Here's how the part is built. I have some questions about the finished solid (model axes, mm). Face numbers are marked on the shaded views. A direction names the side the tool comes from. Coordinates: 2 decimals unless noted, no trailing zeros. Write each loop counter-clockwise with the first axis right and the second up, starting at its lowest first coordinate (ties: lowest second). Pieces come first, ordered by that corner, then holes. Notation, with made-up numbers: (1, 48) -> (5, 48) arc R27 cw to (5, 74) -> close; hole circle Ø5 at (-28.75, -11). An arc over 180 degrees is marked (long way). Use a Markdown table: item, result. Add a question column.
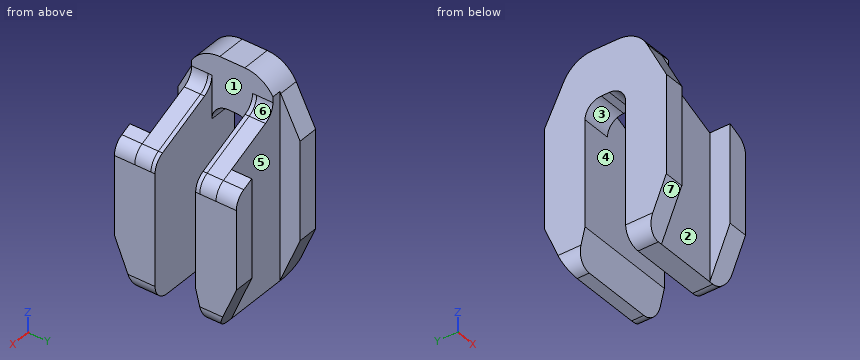
Autodesk Inventor part; units mm, degrees
ref_plane "YZ Plane" through (0, 0, 0) normal (1, 0, 0) x (0, 1, 0)
ref_plane "XZ Plane" through (0, 0, 0) normal (0, 1, 0) x (-1, 0, 0)
ref_plane "XY Plane" through (0, 0, 0) normal (0, 0, 1) x (1, 0, 0)
sketch "Sketch1" plane through (0, 0, 0) normal (0, 0, 1) x (1, 0, 0)
  line L0 (-4.78, -2.9) -> (4.78, -2.9)
  line L1 (6.35, 2.9) -> (-6.35, 2.9)
  line L2 (-4.78, -2.9) -> (-5.08, -2.9)
  line L3 (-6.35, -2.9) -> (-5.08, -2.9)
  line L4 (-6.35, 2.9) -> (-6.35, -2.9)
  line L5 (5.08, -2.9) -> (4.78, -2.9)
  line L6 (5.08, -2.9) -> (6.35, -2.9)
  line L7 (6.35, 3) -> (-6.45, 3)
  line L8 (-6.45, 3) -> (-6.45, -3)
  line L9 (-6.45, -3) -> (-5.08, -3)
  line L10 (-5.08, -3) -> (-4.78, -3)
  line L11 (-4.78, -3) -> (4.78, -3)
  line L12 (4.78, -3) -> (5.08, -3)
  line L13 (5.08, -3) -> (6.35, -3)
  line L14 (6.35, 5) -> (-8.45, 5)
  line L15 (-8.45, 5) -> (-8.45, -5)
  line L16 (-8.45, -5) -> (-5.08, -5)
  line L17 (-5.08, -5) -> (-4.78, -5)
  line L18 (-4.78, -5) -> (4.78, -5)
  line L19 (4.78, -5) -> (5.08, -5)
  line L20 (5.08, -5) -> (6.35, -5)
  line L21 (6.35, 3) -> (6.35, 5)
  line L22 (6.35, -3) -> (6.35, -5)
  point P0 (0, 0)
extrude "Extrusion1" add sketch "Sketch1" against normal blind 2
sketch "Sketch2" plane through (-8.45, -5, 0) normal (0, -1, 0) x (1, 0, 0)
  line L0 (2.1, -8) -> (2.1, -11.17)
  line L1 (0, 0) -> (14.8, 0)
  line L2 (2.1, -8) -> (3.37, -8)
  line L3 (14.8, 0) -> (14.8, -2)
  line L4 (2, 0) -> (14.8, 0)
  line L5 (2, 0) -> (14.8, 0)
  line L6 (14.8, 0) -> (14.8, -8)
  line L7 (14.8, -8) -> (2, -8)
  line L8 (2, -8) -> (2, 0)
  point P0 (8.45, 0)
extrude "Extrusion2" add sketch "Sketch2" against normal up to surface (2 mm away)
sketch "Sketch3" plane through (-8.45, 5, 0) normal (0, 1, 0) x (1, 0, 0)
  line L0 (0, 0) -> (14.8, 0)
  line L1 (0, 0) -> (0, 2)
  line L2 (2, 2) -> (0, 2)
  line L3 (2, 2) -> (2, 8)
  line L4 (2, 8) -> (14.8, 8)
  line L5 (14.8, 0) -> (14.8, 8)
  point P0 (8.45, 0)
extrude "Extrusion3" add sketch "Sketch3" against normal up to surface (2 mm away)
sketch "Sketch4" plane through (-8.45, -5, 0) normal (0, -1, 0) x (1, 0, 0)
  line L0 (2, -2) -> (2, -8)
  line L1 (0, 0) -> (14.8, 0)
  line L2 (3.67, -0.6428) -> (3.67, -14.175)
  line L3 (5.61, -0.6428) -> (5.61, -14.175)
  line L4 (2, -2) -> (5.61, -2)
  line L5 (5.61, -2) -> (5.61, 4)
  line L6 (5.61, 4) -> (2, 4)
  line L7 (2, 4) -> (2, -2)
  point P0 (8.45, 0)
  point P1 (2, 0)
  point P2 (5.61, 0)
  dimension "d8" = 6
extrude "Extrusion4" add sketch "Sketch4" against normal up to surface (10 mm away) contours L7 L6 L5 L1
sketch "Sketch5" plane through (-8.45, -5, -2) normal (0, -1, 0) x (1, 0, 0)
  line L0 (0, 2) -> (0, 0)
  line L1 (0, 2) -> (2, 2)
  line L2 (2, 0) -> (0, 0)
  line L3 (0, 2) -> (2, 2)
  line L4 (2, 2) -> (2, 0)
  line L5 (2, 0) -> (0, 0)
  line L6 (0, 0) -> (0, 2)
  point P0 (8.45, 2)
extrude "Extrusion5" cut sketch "Sketch5" against normal through all
sketch "Sketch6" plane through (-6.45, -5, -8) normal (0, -1, 0) x (1, 0, 0)
  line L0 (3.61, 8) -> (3.61, 12)
  line L1 (3.61, 8) -> (12.8, 8)
  line L2 (3.61, 12) -> (12.8, 8)
  point P0 (6.45, 8)
extrude "Extrusion6" add sketch "Sketch6" against normal up to surface (2 mm away)
sketch "Sketch7" plane through (-6.45, 5, -8) normal (0, 1, 0) x (1, 0, 0)
  line L0 (12.8, -8) -> (3.61, -12)
  line L1 (12.8, -8) -> (3.61, -8)
  line L2 (3.61, -8) -> (3.61, -12)
  point P0 (6.45, -8)
extrude "Extrusion7" add sketch "Sketch7" against normal up to surface (2 mm away)
sketch "Sketch8" plane through (-2.84, -3, 0) normal (1, 0, 0) x (0, 0, -1)
  line L0 (0, 6) -> (-4, 6)
  line L1 (-4, 0) -> (-4, 6)
  line L2 (-4, 0) -> (0, 0)
  line L3 (0, 0) -> (0, 6)
  line L4 (-4, 0) -> (0, 0)
  line L5 (-2, 0) -> (-2, 6)
  point P0 (0, 3)
  point P1 (-2, 0)
extrude "Extrusion8" cut sketch "Sketch8" against normal blind 10 contours L3 L2 L5 L0
sketch "Sketch9" plane through (-6.45, -5, 4) normal (0, 0, 1) x (1, 0, 0)
  line L0 (0, 8) -> (0, 2)
  line L1 (3.61, 10) -> (0, 10)
  line L2 (0, 0) -> (0, 10)
  line L3 (3.61, 0) -> (0, 0)
  line L4 (3.61, 0) -> (3.61, 2)
  line L5 (3.61, 2) -> (3.61, 8)
  line L6 (3.61, 8) -> (3.61, 10)
  point P0 (6.45, 5)
  point P1 (0, 2)
extrude "Extrusion9" add sketch "Sketch9" along normal blind 4
fillet "Fillet1" radius 2 4 edges at (-2.84, 4, 4) (-2.84, -4, 4) (6.35, 4, 0) (6.35, -4, 0)
sketch "Sketch10" plane through (6.35, -5, -8) normal (0, 0, -1) x (-1, 0, 0)
  line L0 (12.8, 2) -> (0, 2)
  line L1 (0, 0) -> (0, 2)
  line L2 (12.8, 0) -> (0, 0)
  line L3 (12.8, 0) -> (12.8, 2)
  line L4 (0, 8) -> (12.8, 8)
  line L5 (12.8, 10) -> (12.8, 8)
  line L6 (0, 10) -> (12.8, 10)
  line L7 (0, 10) -> (0, 8)
  point P0 (6.35, 5)
extrude "Extrusion10" add sketch "Sketch10" along normal blind 4
sketch "Sketch11" plane through (-6.45, 3, 2) normal (0, -1, 0) x (1, 0, 0)
  arc A0 (12.8, -3.3107) -> (11.5982, -1.4769) centre (10.8, -3.3107) ccw
  line L0 (4.8118, 1.4769) -> (11.5982, -1.4769)
  arc A1 (3.61, 3.3107) -> (4.8118, 1.4769) centre (5.61, 3.3107) ccw
  line L1 (3.61, 0) -> (3.61, 3.3107)
  line L2 (3.61, 0) -> (0, 0)
  line L3 (0, 0) -> (0, -14)
  line L4 (12.8, -14) -> (0, -14)
  line L5 (12.8, -3.3107) -> (12.8, -14)
  point P0 (6.45, -2)
extrude "Extrusion11" add sketch "Sketch11" along normal blind 0.5
sketch "Sketch12" plane through (-6.45, -3, 2) normal (0, 1, 0) x (1, 0, 0)
  arc A0 (11.5982, 1.4769) -> (12.8, 3.3107) centre (10.8, 3.3107) ccw
  line L0 (12.8, 3.3107) -> (12.8, 14)
  line L1 (0, 14) -> (12.8, 14)
  line L2 (0, 0) -> (0, 14)
  line L3 (3.61, 0) -> (0, 0)
  line L4 (3.61, -3.3107) -> (3.61, 0)
  arc A1 (4.8118, -1.4769) -> (3.61, -3.3107) centre (5.61, -3.3107) ccw
  line L5 (11.5982, 1.4769) -> (4.8118, -1.4769)
  point P0 (6.45, 2)
extrude "Extrusion12" add sketch "Sketch12" along normal blind 0.5
fillet "Fillet3" radius 2 2 edges at (-4.645, -2.5, 2) (-4.645, 2.5, 2)
sketch "Sketch14" plane through (6.35, -5, -12) normal (0, 0, -1) x (-1, 0, 0)
  line L0 (0, 0) -> (0, 2.5)
  line L1 (0, 0) -> (12.8, 0)
  line L2 (12.8, 0) -> (12.8, 2.5)
  line L3 (0, 2.5) -> (12.8, 2.5)
  line L4 (12.8, 10) -> (12.8, 7.5)
  line L5 (12.8, 10) -> (0, 10)
  line L6 (0, 10) -> (0, 7.5)
  line L7 (12.8, 7.5) -> (0, 7.5)
  point P0 (6.35, 5)
extrude "Extrusion13" add sketch "Sketch14" along normal blind 5
sketch "Sketch15" plane through (6.35, -5, -17) normal (0, 0, -1) x (-1, 0, 0)
  line L0 (12.8, 2.5) -> (0, 2.5)
  line L1 (0, 2.5) -> (0, 0)
  line L2 (0, 0) -> (12.8, 0)
  line L3 (12.8, 0) -> (12.8, 2.5)
  line L4 (0, 7.5) -> (12.8, 7.5)
  line L5 (12.8, 7.5) -> (12.8, 10)
  line L6 (12.8, 10) -> (0, 10)
  line L7 (0, 10) -> (0, 7.5)
  line L8 (12.8, 0) -> (10.3, 0)
  line L9 (10.3, 0) -> (10.3, -2.5)
  line L10 (10.3, -2.5) -> (12.8, -2.5)
  line L11 (12.8, -2.5) -> (12.8, 0)
  line L12 (12.8, 10) -> (10.3, 10)
  line L13 (10.3, 10) -> (10.3, 12.5)
  line L14 (10.3, 12.5) -> (12.8, 12.5)
  line L15 (12.8, 12.5) -> (12.8, 10)
  line L16 (0, 10) -> (2.5, 10)
  line L17 (2.5, 10) -> (2.5, 12.5)
  line L18 (2.5, 12.5) -> (0, 12.5)
  line L19 (0, 12.5) -> (0, 10)
  line L20 (0, 0) -> (2.5, 0)
  line L21 (2.5, 0) -> (2.5, -2.5)
  line L22 (2.5, -2.5) -> (0, -2.5)
  line L23 (0, -2.5) -> (0, 0)
  point P0 (6.35, 5)
  point P1 (2.5, 10)
  point P2 (2.5, 0)
  dimension "d39" = 2.5
  dimension "d40" = 2.5
  dimension "d41" = 2.5
  dimension "d42" = 2.5
  dimension "d43" = 2.5
  dimension "d44" = 2.5
  dimension "d45" = 2.5
  dimension "d46" = 2.5
extrude "Extrusion14" add sketch "Sketch15" against normal up to surface (25 mm away) contours L11 L10 L9 L2 | L2 L21 L22 L23 | L19 L18 L17 L6 | L6 L13 L14 L15
sketch "Sketch16" plane through (3.85, 5, 8) normal (0, -1, 0) x (1, 0, 0)
  line L0 (0, -6.9119) -> (1.2982, -7.4769)
  arc A0 (2.5, -9.3107) -> (1.2982, -7.4769) centre (0.5, -9.3107) ccw
  line L1 (2.5, -9.3107) -> (2.5, 0)
  line L2 (2.5, 0) -> (0, 0)
  line L3 (0, -6.9119) -> (0, 0)
  point P0 (-3.85, -8)
extrude "Extrusion15" cut sketch "Sketch16" along normal mid plane 31
fillet "Fillet5" radius 2 4 edges at (6.35, 5, -17) (-6.45, 5, -17) (6.35, -5, -17) (-6.45, -5, -17)
chamfer "Chamfer3" distance 2.5 angle 45 2 edges at (-5.2, -7.5, 8) (-5.2, 7.5, 8)
sketch "Sketch17" plane through (-6.45, 2.5, -15) normal (-1, 0, 0) x (0, 0, 1)
  line L0 (-2, 5) -> (-2, 0)
  line L1 (-2, 5) -> (0, 5)
  line L2 (0, 5) -> (20.5, 5)
  line L3 (0, 0) -> (-2, 0)
  line L4 (15, 0) -> (0, 0)
  line L5 (-2, 0) -> (-2, 1)
  line L6 (-2, 0) -> (-2, 5)
  line L7 (-2, 0) -> (2, 0)
  line L8 (2, 0) -> (-2, 1)
  point P0 (15, -2.5)
  point P1 (-2, 1)
  dimension "d55" = 1
  dimension "d56" = 4
extrude "Extrusion16" cut sketch "Sketch17" against normal blind 31
sketch "Sketch18" plane through (-6.45, -7.5, -15) normal (-1, 0, 0) x (0, 0, 1)
  line L0 (16.0881, 12.5) -> (-2, 12.5)
  line L1 (0, 15) -> (20.5, 15)
  line L2 (-2, 2.5) -> (16.0881, 2.5)
  line L3 (0, 0) -> (20.5, 0)
  line L4 (-2, 15) -> (0, 15)
  line L5 (-2, 15) -> (-2, 11)
  line L6 (-2, 5) -> (-2, 0)
  line L7 (0, 0) -> (-2, 0)
  line L8 (-2, 0) -> (4, 0)
  line L9 (4, 0) -> (-2, 2.5)
  line L10 (-2, 15) -> (4, 15)
  line L11 (4, 15) -> (-2, 12.5)
  point P0 (15, 7.5)
  dimension "d59" = 6
  dimension "d60" = 6
extrude "Extrusion17" cut sketch "Sketch18" against normal through all
sketch "Sketch19" plane through (-6.45, -2.5, -15) normal (-1, 0, 0) x (0, 0, 1)
  line L0 (23, -2.5) -> (23, 7.5)
  line L1 (20.5, 10) -> (23, 7.5)
  line L2 (23, -2.5) -> (20.5, -5)
  line L3 (4, 10) -> (20.5, 10)
  line L4 (4, -5) -> (20.5, -5)
  line L5 (16.0881, -5) -> (16.0881, -2.5)
  line L6 (16.0881, 7.5) -> (16.0881, 10)
  line L7 (23, -2.5) -> (23, -1.5)
  line L8 (23, -1.5) -> (16.0881, -5)
  line L9 (23, 7.5) -> (23, 6.5)
  line L10 (23, 6.5) -> (16.0881, 10)
  point P0 (15, 2.5)
  dimension "d63" = 1
  dimension "d64" = 1
extrude "Extrusion18" cut sketch "Sketch19" against normal up to surface (3.61 mm away)
fillet "Fillet6" radius 4 2 edges at (-4.645, -4, 8) (-4.645, 4, 8)
properties part number "MolexClipper_vertical_3DPrint"
Q1. Thinking about a two-plate mould opening in Y: for the marked faces 4, 5, 6 and 7, which applies, released by +Y, released by -Y, zero draft, split by the parting line, or undercut?
Q2. Which directions (+Z, -Z, +X, -X, +Y, -Y) give clear straight access to the entire face, cutting with the end or side of a thin tool? Please do the marked faces 1, 2 and 3.
Q3. Suppose I cut it at B-B, the plane z = -6.25. Write out the boundary of the cut face in (x, y), and give its area (3 significant figures).
Q4. Please list where these lines run through material, in increasing order: line 1 (Y direction, x = 0.75, z = -3.25); line 2 (X direction, y = 5.5, z = -7); line 3 (Y direction, x = -4.75, z = -9.75).
Q5. Suppose I cut it at A-A, the plane x = 3.5. Write out the boundary of the cut face in (y, z), and give its area (3 significant figures).
Q6. Will these pins go through, and if not, where does the flat tip stop? pin 1 (2.5 mm diameter, centred on x = -1, z = -0.5, fed in from -Y); pin 2 (4 mm diameter, centred on x = 1.5, z = -1.5, fed in from +Y); pin 3 (1.5 mm diameter, centred on x = 0.5, y = -6, fed in from +Z).
Q7. Suppose I cut it at D-D, the plane z = -12. Write out the boundary of the cut face in (x, y).
Q8. Suppose I cut it at C-C, the plane y = -5.5. Write out the boundary of the cut face in (x, z), and give its area (3 significant figures).
Answer key:
| question | item | result |
|---|---|---|
| 1 | face 4 | undercut |
| 1 | face 5 | released by +Y |
| 1 | face 6 | zero draft |
| 1 | face 7 | released by -Y |
| 2 | face 1 | +Z, +X |
| 2 | face 2 | +Z, -Z, -Y |
| 2 | face 3 | -Z, +X, -X |
| 3 | outline | (-6.45, -7.5) -> (-3.95, -7.5) -> (-3.95, -5) -> (3.85, -5) -> (3.85, -7.5) -> (6.35, -7.5) -> (6.35, -2.5) -> (-6.45, -2.5) -> close; (-6.45, 2.5) -> (6.35, 2.5) -> (6.35, 7.5) -> (3.85, 7.5) -> (3.85, 5) -> (-3.95, 5) -> (-3.95, 7.5) -> (-6.45, 7.5) -> close |
| 3 | area | 89.0 mm^2 |
| 4 | line 1 | y = -5 to -2.5, 2.5 to 5 |
| 4 | line 2 | x = -6.45 to -3.95, 3.85 to 6.35 |
| 4 | line 3 | y = -7.5 to -2.5, 2.5 to 7.5 |
| 5 | outline | (-5, -17) -> (-2.5, -17) -> (-2.5, 1.24) -> (-5, 1.24) -> close; (2.5, -13) -> (3.5, -17) -> (5, -17) -> (5, 1.24) -> (2.5, 1.24) -> close |
| 5 | area | 89.2 mm^2 |
| 6 | pin 1 | stops at y = -5 |
| 6 | pin 2 | stops at y = 5 |
| 6 | pin 3 | passes through |
| 7 | outline | (-6.45, -7.08) -> (-3.95, -7.08) -> (-3.95, -5) -> (3.85, -5) -> (3.85, -7.08) -> (6.35, -7.08) -> (6.35, -2.5) -> (-6.45, -2.5) -> close; (-6.45, 2.5) -> (6.35, 2.5) -> (6.35, 7.08) -> (3.85, 7.08) -> (3.85, 5) -> (-3.95, 5) -> (-3.95, 7.08) -> (-6.45, 7.08) -> close |
| 8 | outline | (-6.45, -15) arc R2 ccw to (-6.28, -15.8) -> (-3.95, -15.8) -> (-3.95, 5.04) -> (-6.45, 5.04) -> close; (3.85, -15.8) -> (6.18, -15.8) arc R2 ccw to (6.35, -15) -> (6.35, -1.31) arc R2 ccw to (5.15, 0.52) -> (3.85, 1.09) -> close |
| 8 | area | 92.6 mm^2 |
